```python
from build123d import *

# Parameters (mm, degrees)
SKETCH1_R           = 18.5
BOSS_EXTRUDE1_DEPTH = 3
SKETCH2_W           = 20.223748417
SKETCH2_H           = 1.96058716
BOSS_EXTRUDE2_DEPTH = 3
CUT_EXTRUDE1_DEPTH  = 3
SKETCH4_W           = 39
SKETCH4_H           = 3
BOSS_EXTRUDE3_DEPTH = 3
CUT_EXTRUDE2_DEPTH  = 3
SKETCH6_R           = 1
CUT_EXTRUDE3_DEPTH  = 3
SKETCH8_W           = 20.223748417
SKETCH8_H           = 50
BOSS_EXTRUDE4_DEPTH = 3


with BuildPart() as part:
    # Sketch1 → Boss-Extrude1 (new body)
    with BuildSketch(Plane(origin=(0, 0, 0), x_dir=(1, 0, 0), z_dir=(0, 1, 0))):
        with Locations(Location((0, 0, 0), (0, 0, 270))):
            Circle(SKETCH1_R)
    extrude(amount=BOSS_EXTRUDE1_DEPTH)

    # Sketch2 → Boss-Extrude2 (add)
    with BuildSketch(Plane.XZ):
        with Locations((0.2001438, 16.339729918)):
            Rectangle(SKETCH2_W, SKETCH2_H)
    extrude(amount=-BOSS_EXTRUDE2_DEPTH)

    # Sketch3 → Cut-Extrude1 (cut)
    with BuildSketch(Plane.XZ):
        with BuildLine():
            Line((6.501291106, 17.320023498), (-6.501291106, 17.320023498))
            ThreePointArc((-6.501291106, 17.320023498), (0, 18.5), (6.501291106, 17.320023498))
        make_face()
    extrude(amount=-CUT_EXTRUDE1_DEPTH, mode=Mode.SUBTRACT)

    # Sketch4 → Boss-Extrude3 (add)
    with BuildSketch(Plane.XZ):
        with Locations((0.200143799, -16.163843272)):
            Rectangle(SKETCH4_W, SKETCH4_H)
    extrude(amount=-BOSS_EXTRUDE3_DEPTH)

    # Sketch5 → Cut-Extrude2 (cut)
    with BuildSketch(Plane.XZ):
        with BuildLine():
            Line((5.498967254, -17.663843272), (-5.498967254, -17.663843272))
            ThreePointArc((-5.498967254, -17.663843272), (0, -18.5), (5.498967254, -17.663843272))
        make_face()
    extrude(amount=-CUT_EXTRUDE2_DEPTH, mode=Mode.SUBTRACT)

    # Sketch6 → Cut-Extrude3 (cut)
    with BuildSketch(Plane.XZ):
        with Locations(Location((17.700143799, -16.163843272, 0), (0, 0, 270))):
            Circle(SKETCH6_R)
        with Locations(Location((-17.700143799, -16.163843272, 0), (0, 0, 270))):
            Circle(SKETCH6_R)
    extrude(amount=-CUT_EXTRUDE3_DEPTH, mode=Mode.SUBTRACT)

    # Sketch8 → Boss-Extrude4 (add)
    with BuildSketch(Plane(origin=(0, 3, 0), x_dir=(1, 0, 0), z_dir=(0, 1, 0))):
        with Locations((0.2001438, -42.320023498)):
            Rectangle(SKETCH8_W, SKETCH8_H)
    extrude(amount=-BOSS_EXTRUDE4_DEPTH)


solid = part.part
```
The model under review builds one solid part; all positions refer to its coordinate system, in mm. A direction names the side the tool comes from. Coordinates: 2 decimals unless noted, no trailing zeros. Write each loop counter-clockwise with the first axis right and the second up, starting at its lowest first coordinate (ties: lowest second). Pieces come first, ordered by that corner, then holes.
1) We need section C-C on x = -12.5. State the section outline as (y, z) points, then the cut area to 3 significant figures.
2) Machinability: for faces 4 (the face through (15, 1, -14.664)), 5 (the face through (10.312, 2, 42)), 6 (the face through (0, 3, 24)), which of the approach directions +Z, -Z, +X, -X, +Y, -Y give a long, thin tool a straight path to every point of the face, cutting with its end or side? Answer none if there is none.
3) Clearance check with flat-ended pins moving along their axes: pin 1 Ø1.2 at (x, z) = (-17.7, -16.16) entering from +Y; pin 2 Ø1.5 at (x, y) = (15, 2.5) entering from +Z; pin 3 Ø1.5 at (y, z) = (2, 34) entering from +X; pin 4 Ø1 at (y, z) = (1, 51.5) entering from -X. State where each tip first meets the part, or that it passes through.
4) We need section D-D on z = 27. State the section outline as (x, y) points.
5) The part is to be moulded in two halves that separate along X. For faces 1 (the face through (17.32, 1.48, -17.09)), 2 (the face through (-15, 1, -14.664)), 3 (the face through (-9.912, 2, 42)), say which applies: pulls with the +X half, pulls with the -X half, needs draft (parallel to the pull), parting line crosses it, or undercut.
6) We need section A-A on x = 14. State the section outline as (y, z) points, then the cut area to 3 significant figures.
7) To check wall thickness, follow probe 1 along X at (y, z) = (2.3, 63); probe 2 along Z at (x, y) = (15, 2.85); probe 3 along X at (y, z) = (1.8, -8). State the ranges of each line that lie inside material, in increasing order.
8) We need section B-B on y = 1.45. State the section outline as (x, z) points.
Answer list:
1. outline: (0, -17.66) - (3, -17.66) - (3, -14.66) - (0, -14.66) - close; (0, -13.64) - (3, -13.64) - (3, 13.64) - (0, 13.64) - close
1. area: 90.8 mm2
2. face 4: +X, +Y, -Y
2. face 5: +Z, +X, +Y, -Y
2. face 6: +Z, -Z, +X, -X, +Y
3. pin 1: passes through
3. pin 2: stops at z = 11.8
3. pin 3: stops at x = 10.31
3. pin 4: stops at x = -9.91
4. outline: (-9.91, 0) - (10.31, 0) - (10.31, 3) - (-9.91, 3) - close
5. face 1: undercut
5. face 2: needs draft
5. face 3: pulls with the -X half
6. outline: (0, -17.66) - (3, -17.66) - (3, -14.66) - (0, -14.66) - close; (0, -12.09) - (3, -12.09) - (3, 12.09) - (0, 12.09) - close
6. area: 81.6 mm2
7. probe 1: x = -9.91 to 10.31
7. probe 2: z = -17.66 to -14.66, -10.83 to 10.83
7. probe 3: x = -16.68 to 16.68
8. outline: (-19.3, -17.66) - (19.7, -17.66) - (19.7, -14.66) - (11.28, -14.66) arc R18.5 ccw to (10.31, 15.36) - (10.31, 67.32) - (-9.91, 67.32) - (-9.91, 15.62) arc R18.5 ccw to (-11.28, -14.66) - (-19.3, -14.66) - close; hole circle Ø2 at (-17.7, -16.16); hole circle Ø2 at (17.7, -16.16)
